Autodesk Inventor part; units mm, degrees
ref_plane "Work Plane1" through (29, 0, 0) normal (0, -1, 0) x (1, 0, 0)
ref_plane "YZ Plane" through (0, 0, 0) normal (1, 0, 0) x (0, 1, 0)
ref_plane "XZ Plane" through (0, 0, 0) normal (0, 1, 0) x (-1, 0, 0)
sketch "Szkic1" plane through (0, 0, 0) normal (0, 0, 1) x (1, 0, 0)
  line L0 (-1.1667, 0) -> (50, 0)
  line L1 (50, 0) -> (50, 2.5)
  line L2 (50, 2.5) -> (28, 2.5)
  line L3 (28, 2.5) -> (27.5091, 2.5)
  line L4 (27.5091, 2.5) -> (0, 2.5)
  line L5 (0, 2.5) -> (0, 4.25)
  line L6 (0, 4.25) -> (-5, 4.25)
  line L7 (-5, 4.25) -> (-5, 2.3094)
  line L8 (-5, 2.3094) -> (-2.5, 2.3094)
  line L9 (-2.5, 2.3094) -> (-1.1667, 0)
  line L10 (-16, 0) -> (61, 0)
  line L11 (0, -0.85) -> (0, 5.1)
  line L12 (28, 2.5) -> (0, 2.5) construction
  dimension "d1" = 22
  dimension "d2" = 0.4909
  dimension "d3" = 5
  dimension "d4" = 2.5
  dimension "d5" = 60
  dimension "d6" = 5
  dimension "d7" = 5
  dimension "d8" = 4.6188
  dimension "d9" = 8.5
  dimension "d26" = 50
revolve "Bryła" add sketch "Szkic1" angle 360 about axis through (-1.1667, 0, 0) along (1, 0, 0)
sketch "Szkic2" plane through (-5, 0, 0) normal (-1, 0, 0) x (0, 0, 1)
  circle A0 centre (0, 0) radius 2.3094
  line L0 (0, -5.95) -> (0, 5.95)
  line L1 (-5.95, 0) -> (5.95, 0)
  line L2 (2.3094, 0) -> (1.1547, -2)
  line L3 (1.1547, -2) -> (-1.1547, -2)
  line L4 (-1.1547, -2) -> (-2.3094, 0)
  line L5 (-2.3094, 0) -> (-1.1547, 2)
  line L6 (-1.1547, 2) -> (1.1547, 2)
  line L7 (1.1547, 2) -> (2.3094, 0)
extrude "Szczelina" add sketch "Szkic2" against normal up to next contours L7 A0 | A0 L2 | L6 L0 A0 | A0 L0 L3 | L0 L6 A0 | A0 L3 L0 | L4 A0 | A0 L5
fillet "Zaokrąglenie1" radius 0.5 1 edges at (-5, -4.25, 0)
thread "Gwint"
chamfer "Faza1" distance 0.4908 distance2 0.4908 1 edges at (50, -2.5, 0) measured on face at (50, -0.1004, 0.8273)
ref_plane "Work Plane1" through (29, 0, 0) normal (0, -1, 0) x (1, 0, 0)
fillet "Fillet2" radius 0.1 1 edges at (0, -2.5, 0)
equation "\"d1\" = GEL"
equation "\"d3\" = KOH"
equation "\"d4\" = INTI"
equation "\"d6\" = GD"
equation "\"d7\" = BDM"
equation "\"d8\" = 1.1547 * SW"
equation "\"d9\" = KOD"
equation "\"d26\" = NLG"
equation "\"d30\" = R"
equation "\"d17\" = RR"
equation "\"d13\" = GEL"
equation "\"d15\" = -0.5 * SPD + 0.5 * GD"
equation "\"d16\" = GUL"
equation "\"GD\" = 5"
equation "\"NLG\" = 50"
equation "\"GEL\" = 22"
equation "\"KOD\" = 8.5"
equation "\"KOH\" = 5"
equation "\"INTI\" = 2.5"
equation "\"GAL\" = 0.61345 * PTC"
equation "\"GUL\" = 0.61345 * PTC"
equation "\"BDM\" = NND"
equation "\"SW\" = 4"
equation "\"RR\" = 0.5"
equation "\"SPD\" = NND - 1.2269 * PTC"
equation "\"R\" = 0.1"
equation "\"TOA\" = 30deg"
equation "\"GD1\" = THREADDIA - 1.2269 * PTC"
equation "\"THREADDIA\" = 5"
equation "\"FAWI\" = 45deg"
equation "\"PTC\" = 0.8"
equation "\"NND\" = 5"
equation "\"E0\" = 1.155 * SW"
properties part number "ISO 4762  - M5 x 50" material "Stal nierdzewna 440C"
Input: part model. Units: mm. Frame: model coordinates. A direction names the side the tool comes from. Round coordinates to 2 decimals unless told otherwise and drop trailing zeros. Order: outer loops, then holes, each group sorted by start corner. A loop starts at its lowest first (then second) coordinate and runs counter-clockwise, first axis right, second up. Notation, with made-up numbers: (-27.75, 2) - (20.25, 2) arc R22 ccw to (20.25, 26) - close; hole circle Ø10 at (-36, 53). An arc over 180 degrees is marked (long way). One line per question, with ' | ' between items. Start each with the question number.
1) Cut plane A-A, the plane x = 5.5. Return the cut outline in (y, z).
2) Pull-direction query (Y, two-part tool) for faces 1 (the flat face through (0, 2, 2)), 2 (the conical face through (-1.25, 0.07, 0.13)), 3 (the cylindrical face through (24.46, -0.54, 2.44)); classes: +Y half, -Y half, draft (parallel to the pull), parting line (faces both ways), or undercut.
3) Ray query, probe 1 along Y at (x, z) = (41, 1.5); probe 2 along X at (y, z) = (-1.75, -2.25); probe 3 along Z at (x, y) = (15, 0). Return the intervals inside material, ascending.
4) Set-up query: faces 4 (the flat face through (-5, -2, 2)), 5 (the flat face through (-4, 2, 0)). Return all of +Z, -Z, +X, -X, +Y, -Y with unobstructed straight access to the full face (end or side cutting, diameter ignored); none if empty.
5) Contact query for flat-ended pins moving along their axis: P1, Ø3, axis at x = 5, z = 0.5, coming from the -Y side; P2, Ø3, axis at x = 39.5, z = -1.5, coming from the +Y side; P3, Ø2, axis at x = 8.5, y = 2, coming from the +Z side; P4, Ø1.2, axis at x = -4, z = 0.5, coming from the +Y side. Output: stop coordinate, or through.
Worked out:
1) outline: circle Ø5 at (0, 0)
2) face 1: draft | face 2: undercut | face 3: parting line
3) probe 1: y = -2 to 2 | probe 2: x = -5 to 0 | probe 3: z = -2.5 to 2.5
4) face 4: +Z, -Z, -X, +Y, -Y | face 5: -X
5) P1: stops at y = -2.5 | P2: stops at y = 2.5 | P3: stops at z = 2.29 | P4: stops at y = 4.25
